Geometry check sheet. Reference: the model listing, model coordinates, mm. A direction names the side the tool comes from. Coordinates: 2 decimals unless noted, no trailing zeros. Write each loop counter-clockwise with the first axis right and the second up, starting at its lowest first coordinate (ties: lowest second). Pieces come first, ordered by that corner, then holes.
from build123d import *

# Parameters (mm, degrees)
F1_DEPTH = 63.5
F0_W     = 25.4
F0_H     = 19.05
F2_DEPTH = 25.4
F3_DEPTH = 7.9375


with BuildPart() as f1:
    # F0 (on Front) → F1 (new body, symmetric)
    with BuildSketch(Plane.XZ):
        Polygon((41.275, -9.525), (41.275, 9.525), (22.225, 9.525), (-41.275, 9.525), (-41.275, -9.525), align=None)
    extrude(amount=F1_DEPTH, both=True)

    # F0 (on Front) → F2 (join, symmetric)
    with BuildSketch(Plane.XZ):
        with BuildLine():
            Line((22.225, 9.525), (41.275, 9.525))
            Line((41.275, 9.525), (41.275, 27.0002))
            ThreePointArc((41.275, 27.0002), (45.9246798487, 38.2255201513), (57.15, 42.8752))
            Line((57.15, 42.8752), (60.325, 42.8752))
            Line((60.325, 42.8752), (60.325, 61.9252))
            Line((60.325, 61.9252), (57.15, 61.9252))
            add(Edge.make_bspline(
                [(57.15, 61.9252), (55.208694365, 61.7794329693), (53.2677947949, 61.6168749598), (51.3302722534, 61.4369012641)],
                knots=[0, 0, 0, 0, 4.4505519897, 4.4505519897, 4.4505519897, 4.4505519897], degree=3))
            ThreePointArc((51.3302722534, 61.4369012641), (30.4759525329, 49.5446187489), (22.225, 27.0002))
            Line((22.225, 27.0002), (22.225, 9.525))
        make_face()
        with Locations((73.025, 52.4002)):
            Rectangle(F0_W, F0_H)
    extrude(amount=F2_DEPTH, both=True)

    # F0 (on Front) → F3 (join, symmetric)
    with BuildSketch(Plane.XZ):
        with BuildLine():
            Line((-41.275, 9.525), (22.225, 9.525))
            Line((22.225, 9.525), (22.225, 27.0002))
            ThreePointArc((22.225, 27.0002), (30.4759525329, 49.5446187489), (51.3302722534, 61.4369012641))
            add(Edge.make_bspline(
                [(51.3302722534, 61.4369012641), (4.7249280234, 57.1077975465), (-39.9264698354, 42.7019898169), (-41.275, 9.525)],
                knots=[4.4505519897, 4.4505519897, 4.4505519897, 4.4505519897, 111.5045361635, 111.5045361635, 111.5045361635, 111.5045361635], degree=3))
        make_face()
    extrude(amount=F3_DEPTH, both=True)

    # F0 (on Front) → F4 (revolve)
    with BuildSketch(Plane.XZ):
        Polygon((85.725, 61.9252), (85.725, 42.8752), (85.725, 38.1), (111.125, 38.1), (111.125, 66.675), (85.725, 66.675), align=None)
    revolve(axis=Axis((85.725, 0, 52.3875), (0, 0, 1)))


solid = f1.part
1. Gauge pin test, flat ends, axial feed: pin 1 Ø8.5 at (y, z) = (17.5, 14) entering from -X (3 decimals); pin 2 Ø1.5 at (x, z) = (56, 44.5) entering from -Y; pin 3 Ø15.5 at (x, z) = (13.5, 38) entering from +Y; pin 4 Ø14 at (y, z) = (-17, 15) entering from -X (3 decimals). Record the tip position at first contact, or that the pin passes through.
Computed values:
pin 1: stops at x = 22.225
pin 2: stops at y = -25.4
pin 3: stops at y = 7.94
pin 4: stops at x = -41.275
2. Access from +Z, -Z, +X, -X, +Y, -Y to the whole of each face (thin tool, end or side, straight path). Record for faces 1 (the cylindrical face through (45.8, -0.4, 38.1)), 2 (the flat face through (22.225, 17, 18)), 3 (the flat face through (60, -2, 61.925)), 4 (the flat face through (46, 25.4, 42)).
Computed values:
face 1: -Z, +Y, -Y
face 2: +Z, -X, +Y
face 3: +Z, -X
face 4: +Z, +X, -X, +Y
3. Thickness scan on line 1 along X through (y, z) = (-57.5, -5.5) (3 decimals); line 2 along Z through (x, y) = (76, -2.5) (3 decimals); line 3 along Z through (x, y) = (-10.5, -55) (3 decimals). Record the ranges inside material, lowest first.
Computed values:
line 1: x = -41.275 to 41.275
line 2: z = 38.1 to 66.675
line 3: z = -9.525 to 9.525
4. Sectioned sample at A-A, the plane y = 28. Record the boundary of the cut face in (x, z) (3 decimals).
Computed values:
outline: (-41.275, -9.525) - (41.275, -9.525) - (41.275, 9.525) - (-41.275, 9.525) - close
5. Draft check along X on faces 5 (the flat face through (22.225, -17, 18)), 6 (the flat face through (60, 2, 42.875)), 7 (the flat face through (-1, -1, -9.525)). Enter one of: released by +X, released by -X, zero draft, split by the parting line, or undercut.
Computed values:
face 5: released by -X
face 6: undercut
face 7: zero draft
